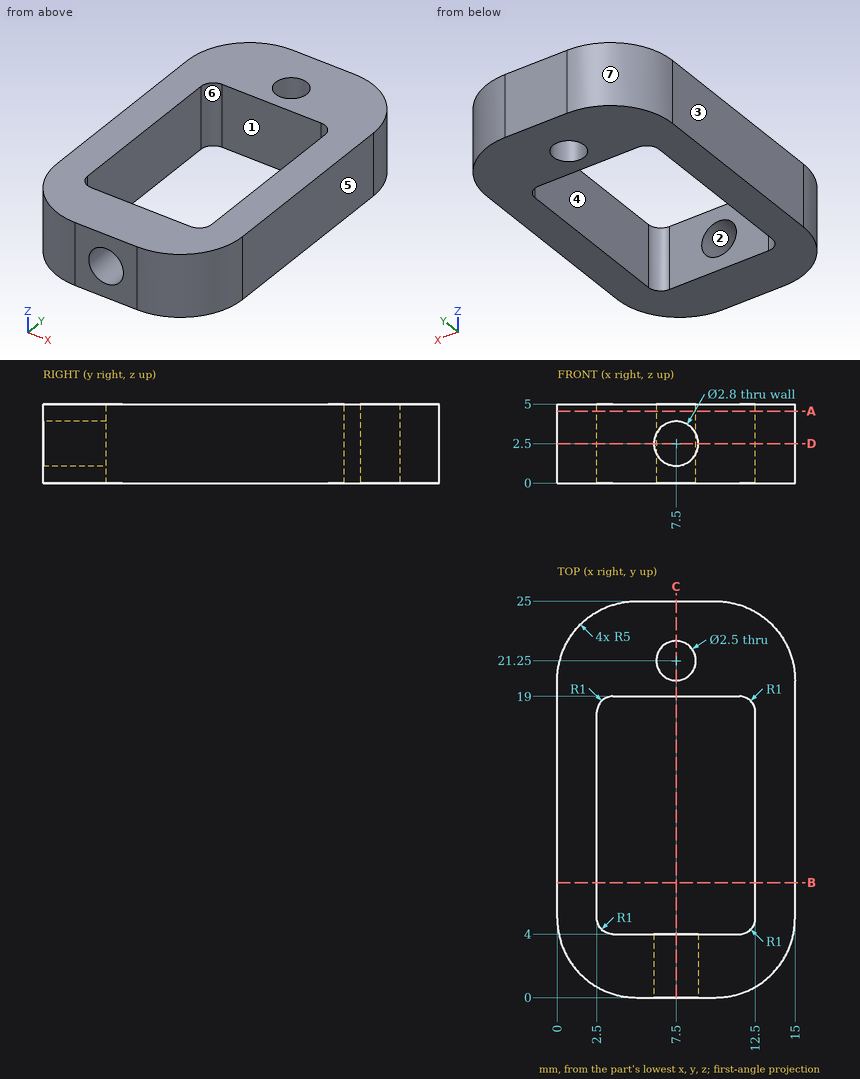
Study the drawing (mm; zero at the part's minimum x, y, z) and answer. A direction names the side the tool comes from. Give positions to 0.01 mm unless a question says otherwise; leave off trailing zeros. Order: outer loops, then holes, each group sorted by start corner. A loop starts at its lowest first (then second) coordinate and runs counter-clockwise, first axis right, second up.
1) Find section D-D on z = 2.5. Write down the section's boundary in (x, y), then the cut area to 3 significant figures.
Reported:
outline: (0, 5) arc R5 ccw to (5, 0) - (6.1, 0) - (6.1, 4) - (3.5, 4) arc R1 cw to (2.5, 5) - (2.5, 18) arc R1 cw to (3.5, 19) - (11.5, 19) arc R1 cw to (12.5, 18) - (12.5, 5) arc R1 cw to (11.5, 4) - (8.9, 4) - (8.9, 0) - (10, 0) arc R5 ccw to (15, 5) - (15, 20) arc R5 ccw to (10, 25) - (5, 25) arc R5 ccw to (0, 20) - close; hole circle Ø2.5 at (7.5, 21.25)
area: 188 mm2
2) Find section C-C on x = 7.5. Write down the section's boundary in (y, z), then the cut area to 3 significant figures.
Reported:
outline: (0, 0) - (4, 0) - (4, 1.1) - (0, 1.1) - close; (0, 3.9) - (4, 3.9) - (4, 5) - (0, 5) - close; (19, 0) - (20, 0) - (20, 5) - (19, 5) - close; (22.5, 0) - (25, 0) - (25, 5) - (22.5, 5) - close
area: 26.3 mm2
3) Given P1, Ø2, axis at y = 21.5, z = 2, coming from the +X side; P2, Ø2, axis at x = 7.5, z = 2.5, coming from the -Y side, each flat-ended and moving along its own axis, determine where each tip first touches the part or whether it passes through.
Reported:
P1: stops at x = 14.97
P2: stops at y = 19
4) Consider line 1 along Y through (x, z) = (5, 1.6); line 2 along Y through (x, z) = (6.5, 4.7); line 3 along X through (y, z) = (13.5, 3.35). Determine where each line is inside the solid, lowest interval first.
Reported:
line 1: y = 0 to 4, 19 to 25
line 2: y = 0 to 4, 19 to 20.5, 22 to 25
line 3: x = 0 to 2.5, 12.5 to 15
5) Determine the mould class of the marked faces 4, 5, 6 and 7 for opening direction X: pulls with the +X half, pulls with the -X half, needs draft (parallel to the pull), parting line crosses it, or undercut.
Reported:
face 4: undercut
face 5: pulls with the +X half
face 6: undercut
face 7: pulls with the -X half
6) For the marked faces 1, 2 and 3, determine the directions among +Z, -Z, +X, -X, +Y, -Y from which every point of the face is accessible in a straight line to the end or side of a thin tool.
Reported:
face 1: +Z, -Z
face 2: -Y
face 3: +Z, -Z, -X, +Y, -Y
7) Find section A-A on z = 4.55. Write down the section's boundary in (x, y).
Reported:
outline: (0, 5) arc R5 ccw to (5, 0) - (10, 0) arc R5 ccw to (15, 5) - (15, 20) arc R5 ccw to (10, 25) - (5, 25) arc R5 ccw to (0, 20) - close; hole (2.5, 5) arc R1 ccw to (3.5, 4) - (11.5, 4) arc R1 ccw to (12.5, 5) - (12.5, 18) arc R1 ccw to (11.5, 19) - (3.5, 19) arc R1 ccw to (2.5, 18) - close; hole circle Ø2.5 at (7.5, 21.25)
8) Find section B-B on y = 7.25. Write down the section's boundary in (x, z), then the cut area to 3 significant figures.
Reported:
outline: (0, 0) - (2.5, 0) - (2.5, 5) - (0, 5) - close; (12.5, 0) - (15, 0) - (15, 5) - (12.5, 5) - close
area: 25.0 mm2
